Check sheet for the modelled part. Datum: model origin and axes. Units: mm. A direction names the side the tool comes from. Coordinates: 2 decimals unless noted, no trailing zeros. Loops run counter-clockwise (first coordinate to the right, second up) from the corner with the lowest first, then second, coordinate; pieces in that order, holes last. Notation, with made-up numbers: (12.25, 79.25) -> (22.25, 79.25) arc R16 cw to (22.25, 84.25) -> close; hole circle Ø4 at (8.5, 77). An arc over 180 degrees is marked (long way). Use CSV: the item, a comma, the result in double quotes. Start each with the question number.
1. Release check for a two-part mould opening along Y. For faces 1 (the face through (190, 0, 6)), 2 (the face through (190, 150.5, 8)), 3 (the face through (190, 81, 0)) record: pulls with the +Y half, pulls with the -Y half, needs draft (parallel to the pull), parting line crosses it, or undercut.
2. Sectioned sample at B-B, the plane x = 176. Record the cut outline in (y, z).
3. Set-up check for faces 4 (the face through (190, 81, 3)), 5 (the face through (178, 9, 13)): record each of +Z, -Z, +X, -X, +Y, -Y from which the full face is reachable in a straight line by a thin tool's end or side.
4. Gauge pin test, flat ends, axial feed: pin 1 (2 mm diameter, centred on x = 370, y = 17, fed in from +Z); pin 2 (1.6 mm diameter, centred on x = 15.5, y = 145, fed in from +Z); pin 3 (6 mm diameter, centred on x = 296.5, y = 106, fed in from -Z). Record the tip position at first contact, or that the pin passes through.
5. Thickness scan on L1, parallel to Y at x = 370, z = 5.3; L2, parallel to X at y = 145, z = 5.2; L3, parallel to Y at x = 5, z = 5.75. Record the ranges inside material, lowest first.
6. Sectioned sample at A-A, the plane y = 25. Record the cut outline in (x, z), and give its area (3 significant figures).
Autodesk Fusion 360 part; units mm, degrees
sketch "Sketch1" plane through (0, 0, 0) normal (0, 0, 1) x (1, 0, 0)
  line L0 (0, 0) -> (385.5, 0)
  line L1 (385.5, 0) -> (385.5, 160.5)
  line L2 (385.5, 160.5) -> (0, 160.5)
  line L3 (0, 160.5) -> (0, 0)
  line L4 (10, 150.5) -> (375.5, 150.5)
  line L5 (375.5, 150.5) -> (375.5, 10)
  line L6 (375.5, 10) -> (10, 10)
  line L7 (10, 10) -> (10, 150.5)
  circle A0 centre (5, 155.5) radius 1.45
  circle A1 centre (5, 5) radius 1.45
  circle A2 centre (380.5, 5) radius 1.45
  circle A3 centre (380.5, 155.5) radius 1.45
  dimension "d1" = 160.5
  dimension "d2" = 385.5
  dimension "d3" = 10
  dimension "d4" = 10
  dimension "d5" = 10
  dimension "d6" = 10
  dimension "d7" = 2.9
  dimension "d8" = 2.9
  dimension "d9" = 2.9
  dimension "d10" = 2.9
  dimension "d11" = 5
  dimension "d12" = 5
  dimension "d13" = 5
  dimension "d14" = 5
  dimension "d15" = 5
  dimension "d16" = 5
  dimension "d17" = 5
  dimension "d18" = 5
extrude "Extrude1" add sketch "Sketch1" along normal blind 13
sketch "Sketch2" plane through (0, 0, 0) normal (0, 0, 1) x (1, 0, 0)
  line L0 (0, 0) -> (385.5, 0)
  line L1 (385.5, 0) -> (385.5, 160.5)
  line L2 (385.5, 160.5) -> (0, 160.5)
  line L3 (0, 160.5) -> (0, 0)
  line L4 (375.5, 10) -> (10, 10)
  line L5 (10, 10) -> (10, 150.5)
  line L6 (10, 150.5) -> (375.5, 150.5)
  line L7 (375.5, 150.5) -> (375.5, 10)
  dimension "d21" = 160.5
  dimension "d22" = 385.5
  dimension "d23" = 10
  dimension "d24" = 10
  dimension "d25" = 365.5
  dimension "d26" = 140.5
extrude "Extrude2" add sketch "Sketch2" along normal blind 3 contours L4 L5 L6 L7
sketch "Sketch3" plane through (0, 0, 0) normal (0, 1, 0) x (1, 0, 0)
sketch "Sketch4" plane through (0, 0, 0) normal (0, 0, 1) x (1, 0, 0)
  line L0 (0, -20) -> (385.5, -20)
  line L1 (385.5, -20) -> (385.5, -180.5)
  line L2 (385.5, -180.5) -> (0, -180.5)
  line L3 (0, -180.5) -> (0, -20)
  line L4 (375.5, -170.5) -> (10, -170.5)
  line L5 (10, -170.5) -> (10, -30)
  line L6 (10, -30) -> (375.5, -30)
  line L7 (375.5, -30) -> (375.5, -170.5)
  circle A0 centre (5, -175.5) radius 1.45
  circle A1 centre (5, -25) radius 1.45
  circle A2 centre (380.5, -25) radius 1.45
  circle A3 centre (380.5, -175.5) radius 1.45
  dimension "d29" = 160.5
  dimension "d30" = 385.5
  dimension "d31" = 10
  dimension "d32" = 10
  dimension "d33" = 10
  dimension "d34" = 10
  dimension "d35" = 2.9
  dimension "d36" = 5
  dimension "d37" = 5
  dimension "d38" = 2.9
  dimension "d39" = 5
  dimension "d40" = 5
  dimension "d41" = 2.9
  dimension "d42" = 5
  dimension "d43" = 5
  dimension "d44" = 2.9
  dimension "d45" = 5
  dimension "d46" = 5
sketch "Sketch5" plane through (0, 0, 3) normal (0, 0, 1) x (-1, 0, 0)
  line L0 (-375.5, -150.5) -> (-10, -150.5)
  line L1 (-10, -150.5) -> (-10, -10)
  line L2 (-10, -10) -> (-375.5, -10)
  line L3 (-375.5, -10) -> (-375.5, -150.5)
  circle A0 centre (-15.5, -145) radius 3.3
  circle A1 centre (-15.5, -145) radius 1.3
  circle A2 centre (-15.5, -15.5) radius 1.3
  circle A3 centre (-15.5, -15.5) radius 3.3
  circle A4 centre (-370, -15.5) radius 1.3
  circle A5 centre (-370, -15.5) radius 3.3
  circle A6 centre (-370, -145) radius 1.3
  circle A7 centre (-370, -145) radius 3.3
  dimension "d49" = 6.6
  dimension "d50" = 5.5
  dimension "d51" = 5.5
  dimension "d52" = 2.6
  dimension "d53" = 2.6
  dimension "d54" = 5.5
  dimension "d55" = 5.5
  dimension "d56" = 6.6
  dimension "d57" = 2.6
  dimension "d58" = 6.6
  dimension "d59" = 5.5
  dimension "d60" = 5.5
  dimension "d61" = 2.6
  dimension "d62" = 6.6
  dimension "d63" = 5.5
  dimension "d64" = 5.5
extrude "Extrude4" add sketch "Sketch5" along normal blind 4 contours A0 | A3 | A5 | A7
sketch "Sketch6" plane through (0, 0, 3) normal (0, 0, 1) x (-1, 0, 0)
  circle A0 centre (-380.5, 25) radius 1.45
sketch "Sketch7" plane through (0, 0, 0) normal (0, 0, -1) x (1, 0, 0)
  circle A0 centre (5, 25) radius 1.45
  circle A1 centre (5, 175.5) radius 1.45
  circle A2 centre (380.5, 25) radius 1.45
  circle A3 centre (380.5, 175.5) radius 1.45
  line L0 (385.5, 180.5) -> (0, 180.5)
  line L1 (0, 180.5) -> (0, 20)
  line L2 (0, 20) -> (385.5, 20)
  line L3 (385.5, 20) -> (385.5, 180.5)
  line L4 (0, 20) -> (385.5, 20)
  line L5 (385.5, 20) -> (385.5, 180.5)
  line L6 (385.5, 180.5) -> (0, 180.5)
  line L7 (0, 180.5) -> (0, 20)
  line L8 (0, 20) -> (385.5, 20)
  line L9 (385.5, 20) -> (385.5, 180.5)
  line L10 (385.5, 180.5) -> (0, 180.5)
  line L11 (0, 180.5) -> (0, 20)
  line L12 (0, 20) -> (385.5, 20)
  line L13 (385.5, 20) -> (385.5, 180.5)
  line L14 (385.5, 180.5) -> (0, 180.5)
  line L15 (0, 180.5) -> (0, 20)
  line L16 (15.5, 165) -> (370, 165)
  line L17 (370, 165) -> (370, 35.5)
  line L18 (370, 35.5) -> (15.5, 35.5)
  line L19 (15.5, 35.5) -> (15.5, 165)
  line L20 (0, 180.5) -> (385.5, 180.5)
  dimension "d68" = 15.5
  dimension "d70" = 15.5
  dimension "d71" = 15.5
  dimension "d72" = 15.5
fillet "Fillet1" radius 4 1 edges at (0, 0, 6.5)
fillet "Fillet2" radius 4 1 edges at (0, 160.5, 6.5)
fillet "Fillet3" radius 4 1 edges at (385.5, 160.5, 6.5)
fillet "Fillet4" radius 4 1 edges at (385.5, 0, 6.5)
Completed:
1,face 1,"pulls with the -Y half"
1,face 2,"undercut"
1,face 3,"needs draft"
2,outline,"(0, 0) -> (160.5, 0) -> (160.5, 13) -> (150.5, 13) -> (150.5, 3) -> (10, 3) -> (10, 13) -> (0, 13) -> close"
3,face 4,"+Z"
3,face 5,"+Z, +X, -X, +Y, -Y"
4,pin 1,"z = 7"
4,pin 2,"z = 3"
4,pin 3,"z = 0"
5,L1,"0 to 10, 12.2 to 14.2, 16.8 to 18.8, 141.7 to 143.7, 146.3 to 148.3, 150.5 to 160.5"
5,L2,"0 to 10, 12.2 to 14.2, 16.8 to 18.8, 366.7 to 368.7, 371.3 to 373.3, 375.5 to 385.5"
5,L3,"0 to 3.55, 6.45 to 154.05, 156.95 to 160.5"
6,outline,"(0, 0) -> (385.5, 0) -> (385.5, 13) -> (375.5, 13) -> (375.5, 3) -> (10, 3) -> (10, 13) -> (0, 13) -> close"
6,area,"1,360 mm²"
